Autodesk Inventor part; units mm, degrees
ref_plane "YZ Plane" through (0, 0, 0) normal (1, 0, 0) x (0, 1, 0)
ref_plane "XZ Plane" through (0, 0, 0) normal (0, 1, 0) x (-1, 0, 0)
ref_plane "XY Plane" through (0, 0, 0) normal (0, 0, 1) x (1, 0, 0)
sketch "Sketch1" plane through (0, 0, 0) normal (0, 0, 1) x (1, 0, 0)
  line L0 (0, 7.4625) -> (0, -7.4625)
  line L1 (-17.6657, 0) -> (17.6657, 0) construction
  line L2 (2, 0.5) -> (5, 0.5)
  line L3 (5, 0.5) -> (5, 0)
  line L4 (5, 0) -> (2, 0)
  line L5 (2, 0) -> (2, 0.5)
  line L6 (3, 0.5) -> (3, 5.5)
  line L7 (3, 5.5) -> (2.9, 5.5)
  line L8 (2.9, 5.5) -> (2, 0.5)
  line L9 (2, -0.5) -> (5, -0.5)
  line L10 (5, -0.5) -> (5, 0)
  line L11 (2, 0) -> (2, -0.5)
  line L12 (3, -0.5) -> (3, -5.5)
  line L13 (3, -5.5) -> (2.9, -5.5)
  line L14 (2.9, -5.5) -> (2, -0.5)
  point P0 (0, 0)
  point P1 (0, 0)
  dimension "d5" = 5
  dimension "d6" = 0.5
  dimension "d7" = 0.1
  dimension "d8" = 6
  dimension "d9" = 1
  dimension "d10" = 10
revolve "Revolution1" add sketch "Sketch1" angle 360 about axis through (0, 7.4625, 0) along (0, -1, 0)
equation "\"d5\" = cn_h"
equation "\"d6\" = 0.5 * w_th"
equation "\"d7\" = tol"
equation "\"d8\" = t_D"
equation "\"d9\" = w_th"
equation "\"d10\" = top_D"
equation "\"tol\" = 0.1"
equation "\"w_th\" = 1"
equation "\"t_D\" = 6"
equation "\"top_D\" = 10"
equation "\"cn_h\" = 5"
equation "\"fillet_D\" = 2"
equation "\"w_l\" = 6"
equation "\"t_D_f\" = t_D + w_th"
equation "\"top_th\" = t_D + w_th"
equation "\"top_th_f\" = t_D_f + cn_h"
equation "\"lv_OD\" = 26"
equation "\"lv_th\" = 1.6"
equation "\"sv_OD\" = 13"
equation "\"sv_th\" = 1.5"
equation "\"b_OD\" = 44"
equation "\"b_th\" = 1.5"
equation "\"b_ID\" = 36.5"
equation "\"b_rim_h\" = 5"
equation "\"h_D\" = 0.9"
equation "\"h_s\" = 2.25"
equation "\"v_h_D\" = 7.5"
equation "\"v_h_off\" = 0.5 * cn_D + 0.5 * v_h_D"
properties part number "adapter"
Read the model definition and answer for the solid it produces. Units are mm, in the model's axes. A direction names the side the tool comes from. Round coordinates to 2 decimals unless told otherwise and drop trailing zeros. Loops run counter-clockwise (first coordinate to the right, second up) from the corner with the lowest first, then second, coordinate; pieces in that order, holes last. Notation, with made-up numbers: (-11.5, 14) - (44.5, 14) arc R26 cw to (44.5, 47) - close; hole circle Ø5 at (60.25, 68.5). An arc over 180 degrees is marked (long way). One line per question, with ' | ' between items. Start each with the question number.
Q1. Section B-B on x = 0 is taken. Give the vertices of the cut face in (y, z).
Q2. Flat-ended cylindrical pins translate along their axes: pin 1 (6 mm diameter, centred on x = 3, z = -2.5, fed in from -Y); pin 2 (1.5 mm diameter, centred on x = 3.5, y = -2, fed in from -Z); pin 3 (5 mm diameter, centred on x = 1, y = 3.5, fed in from +Z); pin 4 (4 mm diameter, centred on y = 4, z = -2.5, fed in from +X). Find the tip coordinate at first contact, or state that the pin passes through.
Q3. Section D-D on x = -4 is taken. Give the vertices of the cut face in (y, z).
Q4. Find the intervals of material crossed by L1, parallel to Z at x = 0, y = 0.25; L2, parallel to Y at x = -2.75, z = -3.5; L3, parallel to X at y = -4.75, z = -0.5, in increasing order.
Q5. Section C-C on y = -4 is taken. Give the vertices of the cut face in (x, z), plus the area to 3 significant figures.
Q6. Section A-A on z = 0 is taken. Give the vertices of the cut face in (x, y), plus the area to 3 significant figures.
Q7. For a pull along Z with two mould halves and no side action, classify faces 4 (the cylindrical face through (-1.08, -0.01, -4.88)), 5 (the flat face through (3.3, 0.5, 0.1)), 6 (the conical face through (2.247, 2.479, -0.708)) as +Z half, -Z half, draft (parallel to the pull), parting line (faces both ways), or undercut.
Q8. For faces 1 (the cylindrical face through (0, 0, -2)), 2 (the cylindrical face through (-3, 3, 0)), 3 (the flat face through (3.3, -0.5, 0.1)), determine the directions among +Z, -Z, +X, -X, +Y, -Y from which every point of the face is accessible in a straight line to the end or side of a thin tool.
Established:
1) outline: (-5.5, -3) - (-0.5, -3) - (-0.5, -5) - (0.5, -5) - (0.5, -3) - (5.5, -3) - (5.5, -2.9) - (0.5, -2) - (-0.5, -2) - (-5.5, -2.9) - close; (-5.5, 2.9) - (-0.5, 2) - (0.5, 2) - (5.5, 2.9) - (5.5, 3) - (0.5, 3) - (0.5, 5) - (-0.5, 5) - (-0.5, 3) - (-5.5, 3) - close
2) pin 1: y = -5.5 | pin 2: z = -1.2 | pin 3: z = 3 | pin 4: x = 2.96
3) outline: (-0.5, -3) - (0.5, -3) - (0.5, 3) - (-0.5, 3) - close
4) L1: -5 to -2, 2 to 5 | L2: -0.5 to 0.5 | L3: -2.96 to -2.72, 2.72 to 2.96
5) outline: circle Ø6 at (0, 0); hole circle Ø5.26 at (0, 0) | area: 6.54 mm²
6) outline: (-5, -0.5) - (-3, -0.5) - (-3, -5.5) - (-2.9, -5.5) - (-2, -0.5) - (-2, 0.5) - (-2.9, 5.5) - (-3, 5.5) - (-3, 0.5) - (-5, 0.5) - close; (2, -0.5) - (2.9, -5.5) - (3, -5.5) - (3, -0.5) - (5, -0.5) - (5, 0.5) - (3, 0.5) - (3, 5.5) - (2.9, 5.5) - (2, 0.5) - close | area: 17.0 mm²
7) face 4: parting line | face 5: draft | face 6: undercut
8) face 1: +Y, -Y | face 2: +Y | face 3: -Y
